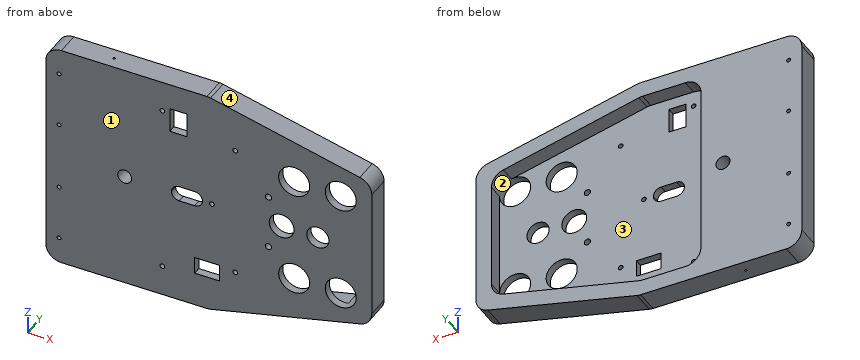
from build123d import *

# Parameters (mm, degrees)
ESBO_O1_R                = 4.5
ESBO_O1_R_2              = 7.14
ESBO_O1_R_3              = 8
ESBO_O1_R_4              = 1.25
RESSALTO_EXTRUS_O1_DEPTH = 15
CORTE_EXTRUS_O2_DEPTH    = 10
FILETE1_R                = 10
ESBO_O5_R                = 2
ESBO_O5_W                = 20
ESBO_O5_H                = 10
CORTE_EXTRUS_O4_DEPTH    = 224.494966386
FILETE2_R                = 5
ESBO_O6_R                = 10
CORTE_EXTRUS_O5_DEPTH    = 224.494966386
ESBO_O7_W                = 11
ESBO_O7_H                = 16
ESBO_O7_W_2              = 16
ESBO_O7_H_2              = 11
ESBO_O7_R                = 1.5
CORTE_EXTRUS_O6_DEPTH    = 224.494966386
ESBO_O8_R                = 0.75
CORTE_EXTRUS_O7_DEPTH    = 259.505319094


with BuildPart() as part:
    # Esboço1 → Ressalto-extrusão1 (new body)
    with BuildSketch(Plane(origin=(0, 0, 0), x_dir=(1, 0, 0), z_dir=(0, 1, 0))):
        Polygon((210, 50), (105, 75), (0, 75), (0, -75), (105, -75), (210, -50), align=None)
        with Locations(Location((50.8, 0, 0), (0, 0, 270))):
            Circle(ESBO_O1_R, mode=Mode.SUBTRACT)
        with Locations(Location((175.26, 0, 0), (0, 0, 270))):
            Circle(ESBO_O1_R_2, mode=Mode.SUBTRACT)
        with Locations(Location((151.92, 0, 0), (0, 0, 270))):
            Circle(ESBO_O1_R_3, mode=Mode.SUBTRACT)
        with Locations(Location((8.5, -58, 0), (0, 0, 270))):
            Circle(ESBO_O1_R_4, mode=Mode.SUBTRACT)
        with Locations(Location((8.5, -22, 0), (0, 0, 270))):
            Circle(ESBO_O1_R_4, mode=Mode.SUBTRACT)
        with Locations(Location((8.5, 22, 0), (0, 0, 90))):
            Circle(ESBO_O1_R_4, mode=Mode.SUBTRACT)
        with Locations(Location((8.5, 58, 0), (0, 0, 90))):
            Circle(ESBO_O1_R_4, mode=Mode.SUBTRACT)
    extrude(amount=RESSALTO_EXTRUS_O1_DEPTH)

    # Esboço3 → Corte-extrusão2 (cut)
    with BuildSketch(Plane(origin=(0, 15, 0), x_dir=(1, 0, 0), z_dir=(0, 1, 0))):
        Polygon((200, 42.101412788), (200, -42.101412788), (103.82593371, -65), (65, -65), (65, 65), (103.82593371, 65), align=None)
    extrude(amount=-CORTE_EXTRUS_O2_DEPTH, mode=Mode.SUBTRACT)

    # Filete1
    filete1_edges = [part.edges().sort_by_distance(p)[0] for p in [
        (0, 7.5, -75),
        (105, 7.5, -75),
        (210, 7.5, -50),
        (210, 7.5, 50),
        (105, 7.5, 75),
        (0, 7.5, 75),
        (65, 10, 65),
        (65, 10, -65),
        (103.82593371, 10, -65),
        (200, 10, -42.101412788),
        (200, 10, 42.101412788),
        (103.82593371, 10, 65),
    ]]
    fillet(filete1_edges, radius=FILETE1_R)

    # Esboço5 → Corte-extrusão4 (cut, through all)
    with BuildSketch(Plane.XZ):
        with Locations(Location((143.42, 17.5, 0), (0, 0, 270))):
            Circle(ESBO_O5_R)
        with Locations(Location((143.42, -17.5, 0), (0, 0, 270))):
            Circle(ESBO_O5_R)
        with Locations((90.92, 0)):
            Rectangle(ESBO_O5_W, ESBO_O5_H)
    extrude(amount=-CORTE_EXTRUS_O4_DEPTH, mode=Mode.SUBTRACT)

    # Filete2
    filete2_edges = [part.edges().sort_by_distance(p)[0] for p in [
        (80.92, 2.5, -5),
        (80.92, 2.5, 5),
        (100.92, 2.5, 5),
        (100.92, 2.5, -5),
    ]]
    fillet(filete2_edges, radius=FILETE2_R - 0.0001)  # a hair under: the kernel refuses the full size

    # Esboço6 → Corte-extrusão5 (cut, through all)
    with BuildSketch(Plane(origin=(0, 15, 0), x_dir=(1, 0, 0), z_dir=(0, 1, 0))):
        with Locations(Location((190, -34.202825576, 0), (0, 0, 270))):
            Circle(ESBO_O6_R)
        with Locations(Location((190, 34.202825576, 0), (0, 0, 90))):
            Circle(ESBO_O6_R)
        with Locations(Location((160, 34.202825576, 0), (0, 0, 270))):
            Circle(ESBO_O6_R)
        with Locations(Location((160, -34.202825576, 0), (0, 0, 270))):
            Circle(ESBO_O6_R)
    extrude(amount=-CORTE_EXTRUS_O5_DEPTH, mode=Mode.SUBTRACT)

    # Esboço7 → Corte-extrusão6 (cut, through all)
    with BuildSketch(Plane.XZ):
        with Locations((85.4, 50.1)):
            Rectangle(ESBO_O7_W, ESBO_O7_H)
        with Locations((103.9, -47.2)):
            Rectangle(ESBO_O7_W_2, ESBO_O7_H_2)
        with Locations(Location((75, 55, 0), (0, 0, 270))):
            Circle(ESBO_O7_R)
        with Locations(Location((122, 43, 0), (0, 0, 270))):
            Circle(ESBO_O7_R)
        with Locations(Location((107, 0, 0), (0, 0, 270))):
            Circle(ESBO_O7_R)
        with Locations(Location((75, -55, 0), (0, 0, 270))):
            Circle(ESBO_O7_R)
        with Locations(Location((122, -43, 0), (0, 0, 270))):
            Circle(ESBO_O7_R)
    extrude(amount=-CORTE_EXTRUS_O6_DEPTH, mode=Mode.SUBTRACT)

    # Esboço8 → Corte-extrusão7 (cut, through all)
    with BuildSketch(Plane.XY.offset(75)):
        with Locations((40, 7.5)):
            Circle(ESBO_O8_R)
    extrude(amount=-CORTE_EXTRUS_O7_DEPTH, mode=Mode.SUBTRACT)


solid = part.part
Model file for the job. Use its own axes, mm. Face numbers are marked on the shaded views. Round coordinates to 2 decimals unless told otherwise and drop trailing zeros. Order: outer loops, then holes, each group sorted by start corner. A loop starts at its lowest first (then second) coordinate and runs counter-clockwise, first axis right, second up. Notation, with made-up numbers: M 26,6.5 L 76,6.5 A5 cw 76,12.5 Z; hole C 13.5,14.25 d5. An arc over 180 degrees is marked long. Write each question's results on one line, items separated by ' | '. Start each with the question number.
(1) Saw through at A-A, the plane y = 10.5. State how many separate pieces and enclosed holes the cut face has, then the cut area to 3 significant figures.
(2) Saw through at B-B, the plane z = 39. Give the cut face in (x, y), then the cut area to 3 significant figures.
(3) Two-plate mould, pull along X, no slides. Class the marked faces 1, 2, 3 and 4: pulls with the +X half, pulls with the -X half, needs draft (parallel to the pull), parting line crosses it, or undercut.
(4) Saw through at D-D, the plane x = 116. Give the cut face in (y, z), then the cut area to 3 significant figures.
(5) Probe probe 1 along X at (y, z) = (1.8, 0); probe 2 along Y at (x, z) = (40, 40); probe 3 along Z at (x, y) = (80.5, 9.25). List the from-to ranges inside material, lowest first. Write a range as from..to.
(6) Saw through at C-C, the plane x = 175.26. Give the cut face in (y, z), then the cut area to 3 significant figures.
(7) Drop flat-ended pins along their axis: pin 1 (1.5 mm diameter, centred on x = 116.5, z = -51.5, fed in from +Y); pin 2 (1.5 mm diameter, centred on y = 3, z = 47, fed in from +X). Give the stop position or say it passes through.
Established:
1) separate pieces: 1 | enclosed holes: 6 | area: 13,400 mm^2
2) outline: M 0,0 L 151.23,0 L 151.23,5 L 65,5 L 65,15 L 0,15 Z; M 168.77,0 L 181.23,0 L 181.23,5 L 168.77,5 Z; M 198.77,0 L 210,0 L 210,15 L 198.77,15 Z; hole C 40,7.5 d1.5 | area: 1,640 mm^2
3) face 1: needs draft | face 2: undercut | face 3: undercut | face 4: pulls with the +X half
4) outline: M 0,-72.38 L 15,-72.38 L 15,-62.1 L 5,-62.1 L 5,62.1 L 15,62.1 L 15,72.38 L 0,72.38 Z | area: 929 mm^2
5) probe 1: x = 0..46.3, 55.3..80.92, 100.92..105.5, 108.5..143.92, 159.92..168.12, 182.4..210 | probe 2: y = 0..6.75, 8.25..15 | probe 3: z = -75..-65, 65..75
6) outline: M 0,-58.27 L 15,-58.27 L 15,-47.99 L 5,-47.99 L 5,-7.14 L 0,-7.14 Z; M 0,7.14 L 5,7.14 L 5,47.99 L 15,47.99 L 15,58.27 L 0,58.27 Z | area: 717 mm^2
7) pin 1: stops at y = 5 | pin 2: stops at x = 209.1
